```python
from build123d import *

# Parameters (mm, degrees)
LID_PLATE_START                    = 32.5
LID_FOOTPRINT_W                    = 134.2
LID_FOOTPRINT_H                    = 68.4
LID_PLATE_DEPTH                    = 3
WHEEL_CLEARANCE_WINDOWS_START      = 36
WHEEL_WELL_PROFILE_W               = 21.2
WHEEL_WELL_PROFILE_H               = 46.2
WHEEL_CLEARANCE_WINDOWS_DEPTH      = 5
LID_STIFFENING_RIBS_START          = 29.5
LID_RIB_PROFILE_W                  = 78
LID_RIB_PROFILE_H                  = 2.5
LID_STIFFENING_RIBS_DEPTH          = 3
LID_MOTOR_CLAMP_BLOCKS_START       = 23.6
UPPER_MOTOR_CLAMP_PROFILE_W        = 10
UPPER_MOTOR_CLAMP_PROFILE_H        = 19
LID_MOTOR_CLAMP_BLOCKS_DEPTH       = 8.9
UPPER_MOTOR_CLAMP_SEATS_R8P2_START = 36
UPPER_CLAMP_RADIUS_PROFILE_R       = 8.2
UPPER_MOTOR_CLAMP_SEATS_R8P2_DEPTH = 72
REGISTRATION_TABS_START            = 31
LID_REGISTRATION_PROFILE_W         = 32
LID_REGISTRATION_PROFILE_H         = 0.9
REGISTRATION_TABS_DEPTH            = 1.5
BATTERY_SOFT_PAD_STOPS_START       = 21.1
BATTERY_UPPER_STOP_PROFILE_W       = 8
BATTERY_UPPER_STOP_PROFILE_H       = 8
BATTERY_SOFT_PAD_STOPS_DEPTH       = 11.4
LID_M3_CLEARANCE_HOLES_START       = 36
LID_M3_CLEARANCE_PROFILE_R         = 1.7
LID_M3_CLEARANCE_HOLES_DEPTH       = 5
SWITCH_RETENTION_RAILS_START       = 18.4
SWITCH_RETENTION_RAIL_PROFILE_W    = 1.7
SWITCH_RETENTION_RAIL_PROFILE_H    = 8.3
SWITCH_RETENTION_RAILS_DEPTH       = 14.1
SWITCH_RETENTION_LEDGES_START      = 17.4
SWITCH_RETENTION_LEDGE_PROFILE_W   = 2.7
SWITCH_RETENTION_LEDGE_PROFILE_H   = 8.3
SWITCH_RETENTION_LEDGES_DEPTH      = 1
SWITCH_TOOL_ACCESS_START           = 36
SWITCH_TOOL_ACCESS_PROFILE_R       = 3.25
SWITCH_TOOL_ACCESS_DEPTH           = 5
LID_OUTER_CORNERS_R4_R             = 4
SNAKE_LOGO_ENGRAVED_START          = 35.5
SNAKE_LOGO_ENGRAVED_DEPTH          = 0.4


with BuildPart() as part:
    # Lid_Footprint → Lid_Plate (new body)
    with BuildSketch(Plane.XY.offset(LID_PLATE_START)):
        Rectangle(LID_FOOTPRINT_W, LID_FOOTPRINT_H)
    extrude(amount=LID_PLATE_DEPTH)

    # Wheel_Well_Profile → Wheel_Clearance_Windows (cut)
    with BuildSketch(Plane.XY.offset(WHEEL_CLEARANCE_WINDOWS_START)):
        with Locations((53.5, 0)):
            Rectangle(WHEEL_WELL_PROFILE_W, WHEEL_WELL_PROFILE_H)
        with Locations((-53.5, 0)):
            Rectangle(WHEEL_WELL_PROFILE_W, WHEEL_WELL_PROFILE_H)
    extrude(amount=-WHEEL_CLEARANCE_WINDOWS_DEPTH, mode=Mode.SUBTRACT)

    # Lid_Rib_Profile → Lid_Stiffening_Ribs (add)
    with BuildSketch(Plane.XY.offset(LID_STIFFENING_RIBS_START)):
        with Locations((0, -6.75)):
            Rectangle(LID_RIB_PROFILE_W, LID_RIB_PROFILE_H)
        with Locations((0, 6.75)):
            Rectangle(LID_RIB_PROFILE_W, LID_RIB_PROFILE_H)
    extrude(amount=LID_STIFFENING_RIBS_DEPTH)

    # Upper_Motor_Clamp_Profile → Lid_Motor_Clamp_Blocks (add)
    with BuildSketch(Plane.XY.offset(LID_MOTOR_CLAMP_BLOCKS_START)):
        with Locations((-30.1, 0)):
            Rectangle(UPPER_MOTOR_CLAMP_PROFILE_W, UPPER_MOTOR_CLAMP_PROFILE_H)
        with Locations((30.1, 0)):
            Rectangle(UPPER_MOTOR_CLAMP_PROFILE_W, UPPER_MOTOR_CLAMP_PROFILE_H)
    extrude(amount=LID_MOTOR_CLAMP_BLOCKS_DEPTH)

    # Upper_Clamp_Radius_Profile → Upper_Motor_Clamp_Seats_R8p2 (cut)
    with BuildSketch(Plane(origin=(0, 0, 0), x_dir=(0, 0, -1), z_dir=(1, 0, 0)).offset(UPPER_MOTOR_CLAMP_SEATS_R8P2_START)):
        with Locations((-19.6, 0)):
            Circle(UPPER_CLAMP_RADIUS_PROFILE_R)
    extrude(amount=-UPPER_MOTOR_CLAMP_SEATS_R8P2_DEPTH, mode=Mode.SUBTRACT)

    # Lid_Registration_Profile → Registration_Tabs (add)
    with BuildSketch(Plane.XY.offset(REGISTRATION_TABS_START)):
        with Locations((-16.5, 30.45)):
            Rectangle(LID_REGISTRATION_PROFILE_W, LID_REGISTRATION_PROFILE_H)
        with Locations((16.5, 30.45)):
            Rectangle(LID_REGISTRATION_PROFILE_W, LID_REGISTRATION_PROFILE_H)
        with Locations((-16.5, -30.45)):
            Rectangle(LID_REGISTRATION_PROFILE_W, LID_REGISTRATION_PROFILE_H)
        with Locations((16.5, -30.45)):
            Rectangle(LID_REGISTRATION_PROFILE_W, LID_REGISTRATION_PROFILE_H)
    extrude(amount=REGISTRATION_TABS_DEPTH)

    # Battery_Upper_Stop_Profile → Battery_Soft_Pad_Stops (add)
    with BuildSketch(Plane.XY.offset(BATTERY_SOFT_PAD_STOPS_START)):
        with Locations((-11, 21)):
            Rectangle(BATTERY_UPPER_STOP_PROFILE_W, BATTERY_UPPER_STOP_PROFILE_H)
        with Locations((11, 21)):
            Rectangle(BATTERY_UPPER_STOP_PROFILE_W, BATTERY_UPPER_STOP_PROFILE_H)
    extrude(amount=BATTERY_SOFT_PAD_STOPS_DEPTH)

    # Lid_M3_Clearance_Profile → Lid_M3_Clearance_Holes (cut)
    with BuildSketch(Plane.XY.offset(LID_M3_CLEARANCE_HOLES_START)):
        with Locations(Location((-52, -28.5, 0), (0, 0, 180))):
            Circle(LID_M3_CLEARANCE_PROFILE_R)
        with Locations(Location((-52, 28.5, 0), (0, 0, 180))):
            Circle(LID_M3_CLEARANCE_PROFILE_R)
        with Locations(Location((52, -28.5, 0), (0, 0, 180))):
            Circle(LID_M3_CLEARANCE_PROFILE_R)
        with Locations(Location((52, 28.5, 0), (0, 0, 180))):
            Circle(LID_M3_CLEARANCE_PROFILE_R)
    extrude(amount=-LID_M3_CLEARANCE_HOLES_DEPTH, mode=Mode.SUBTRACT)

    # Switch_Retention_Rail_Profile → Switch_Retention_Rails (add)
    with BuildSketch(Plane.XY.offset(SWITCH_RETENTION_RAILS_START)):
        with Locations((-10.65, -14.35)):
            Rectangle(SWITCH_RETENTION_RAIL_PROFILE_W, SWITCH_RETENTION_RAIL_PROFILE_H)
        with Locations((10.65, -14.35)):
            Rectangle(SWITCH_RETENTION_RAIL_PROFILE_W, SWITCH_RETENTION_RAIL_PROFILE_H)
    extrude(amount=SWITCH_RETENTION_RAILS_DEPTH)

    # Switch_Retention_Ledge_Profile → Switch_Retention_Ledges (add)
    with BuildSketch(Plane.XY.offset(SWITCH_RETENTION_LEDGES_START)):
        with Locations((-10.15, -14.35)):
            Rectangle(SWITCH_RETENTION_LEDGE_PROFILE_W, SWITCH_RETENTION_LEDGE_PROFILE_H)
        with Locations((10.15, -14.35)):
            Rectangle(SWITCH_RETENTION_LEDGE_PROFILE_W, SWITCH_RETENTION_LEDGE_PROFILE_H)
    extrude(amount=SWITCH_RETENTION_LEDGES_DEPTH)

    # Switch_Tool_Access_Profile → Switch_Tool_Access (cut)
    with BuildSketch(Plane.XY.offset(SWITCH_TOOL_ACCESS_START)):
        with Locations(Location((3.175, -14.325, 0), (0, 0, 180))):
            Circle(SWITCH_TOOL_ACCESS_PROFILE_R)
    extrude(amount=-SWITCH_TOOL_ACCESS_DEPTH, mode=Mode.SUBTRACT)

    # Lid_Outer_Corners_R4
    lid_outer_corners_r4_edges = [part.edges().sort_by_distance(p)[0] for p in [
        (-67.1, 34.2, 34),
        (67.1, 34.2, 34),
        (67.1, -34.2, 34),
        (-67.1, -34.2, 34),
    ]]
    fillet(lid_outer_corners_r4_edges, radius=LID_OUTER_CORNERS_R4_R)

    # Snake_Logo_Native_Profile → Snake_Logo_Engraved (cut)
    # profile 1 of 2: a face of its own
    with BuildSketch(Plane.XY.offset(SNAKE_LOGO_ENGRAVED_START)):
        Polygon((13.800582242, 26.557496361), (14.851528384, 25.064046579), (14.851528384, 24.898107715), (6.443959243, 19.311499272), (14.243085881, 18.703056769), (15.459970888, 22.851528384), (15.625909753, 23.349344978), (15.791848617, 23.459970888), (19, 17.983988355), (9.430858806, 12.010189229), (4.397379913, -0.767103348), (4.065502183, -1.320232897), (5.890829694, 11.45705968), (0.027656477, 13.890829694), (-5.890829694, 11.45705968), (-4.065502183, -0.877729258), (-4.065502183, -1.264919942), (-4.176128093, -1.320232897), (-9.430858806, 12.010189229), (-19, 17.983988355), (-15.791848617, 23.459970888), (-15.570596798, 23.183406114), (-14.243085881, 18.703056769), (-6.443959243, 19.311499272), (-14.851528384, 24.898107715), (-14.851528384, 25.064046579), (-13.911208151, 26.502183406), (-0.414847162, 24.84279476), (0.414847162, 24.84279476), align=None)
        Polygon((-4.452692868, 14.720524017), (-2.018922853, 14.775836972), (-3.788937409, 16.490538574), align=None, mode=Mode.SUBTRACT)
        Polygon((1.963609898, 14.720524017), (4.452692868, 14.720524017), (3.788937409, 16.490538574), align=None, mode=Mode.SUBTRACT)
    # profile 2 of 2: a face of its own
    with BuildSketch(Plane.XY.offset(SNAKE_LOGO_ENGRAVED_START)):
        Polygon((-16.84279476, 15.107714702), (-16.566229985, 15.052401747), (-16.62154294, 14.941775837), (-16.510917031, 14.997088792), (-15.902474527, 14.554585153), (-13.136826783, 12.397379913), (-13.026200873, 12.176128093), (-6.775836972, -5.855895197), (-3.788937409, -6.740902475), (-3.180494905, -4.141193595), (-3.014556041, -4.08588064), (-2.240174672, -7.183406114), (-0.082969432, -7.847161572), (2.240174672, -7.128093159), (3.014556041, -4.141193595), (3.180494905, -4.19650655), (3.788937409, -6.740902475), (6.775836972, -5.855895197), (13.081513828, 12.342066958), (16.62154294, 15.107714702), (16.787481805, 14.997088792), (13.800582242, 12.010189229), (7.937409025, -7.625909753), (0.304221252, -10.502183406), (-0.138282387, -10.557496361), (-7.937409025, -7.625909753), (-13.800582242, 12.010189229), align=None)
    extrude(amount=-SNAKE_LOGO_ENGRAVED_DEPTH, mode=Mode.SUBTRACT)


solid = part.part
```
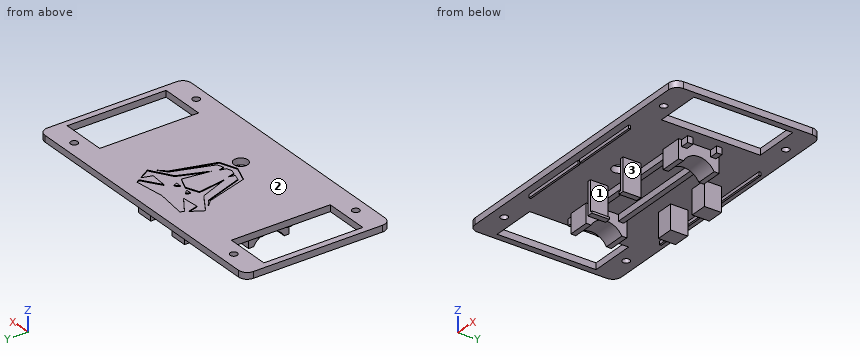
The model under review builds one solid part; all positions refer to its coordinate system, in mm. Face numbers are marked on the shaded views. Round coordinates to 2 decimals unless told otherwise and drop trailing zeros. Loops run counter-clockwise (first coordinate to the right, second up) from the corner with the lowest first, then second, coordinate; pieces in that order, holes last. Notation, with made-up numbers: (-25, -39) - (29, -39) arc R27 cw to (29, -9) - close; hole circle Ø6 at (-38.75, 4). An arc over 180 degrees is marked (long way). Use a Markdown table: item, result. Add a question column.
Q1. Add section D-D (x = -47.5). State the section outline as (y, z) points, plus the area to 3 significant figures.
Q2. For probe 1 along X at (y, z) = (28.5, 33.85); probe 2 along X at (y, z) = (3, 34.5); probe 3 along Y at (x, z) = (-52, 33.7), list the stretches that pass through material, from the lowest coordinate up.
Q3. Insertion check: pin 1 Ø1.2 at (x, z) = (17, 32) entering from -Y; pin 2 Ø0.8 at (x, z) = (-14.5, 31.5) entering from +Y; pin 3 Ø5 at (x, y) = (-10, 15.5) entering from +Z; pin 4 Ø2 at (x, y) = (36, 7) entering from -Z. Each pin has a flat end and moves straight along its axis. Give the tip position at first contact, or say it passes through.
Q4. Add section C-C (x = 23.5). State the section outline as (y, z) points, plus the area to 3 significant figures.
Q5. Add section A-A (y = -28.5). State the section outline as (x, z) points.
Q6. The part is to be moulded in two halves that separate along X. For the marked faces 1, 2 and 3, say which applies: pulls with the +X half, pulls with the -X half, needs draft (parallel to the pull), parting line crosses it, or undercut.
Q7. Add section B-B (x = 52). State the section outline as (y, z) points.
Worked answers:
| question | item | result |
|---|---|---|
| 1 | outline | (-34.2, 32.5) - (-23.1, 32.5) - (-23.1, 35.5) - (-34.2, 35.5) - close; (23.1, 32.5) - (34.2, 32.5) - (34.2, 35.5) - (23.1, 35.5) - close |
| 1 | area | 66.6 mm² |
| 2 | probe 1 | -67.1 to -53.7, -50.3 to 50.3, 53.7 to 67.1 |
| 2 | probe 2 | -67.1 to -64.1, -42.9 to 42.9, 64.1 to 67.1 |
| 2 | probe 3 | -34.2 to -30.2, -26.8 to -23.1, 23.1 to 26.8, 30.2 to 34.2 |
| 3 | pin 1 | y = -34.2 |
| 3 | pin 2 | y = 30.9 |
| 3 | pin 3 | z = 35.1 |
| 3 | pin 4 | z = 23.6 |
| 4 | outline | (-34.2, 32.5) - (-30.9, 32.5) - (-30.9, 31) - (-30, 31) - (-30, 32.5) - (-8, 32.5) - (-8, 29.5) - (-5.5, 29.5) - (-5.5, 32.5) - (5.5, 32.5) - (5.5, 29.5) - (8, 29.5) - (8, 32.5) - (30, 32.5) - (30, 31) - (30.9, 31) - (30.9, 32.5) - (34.2, 32.5) - (34.2, 35.5) - (-34.2, 35.5) - close |
| 4 | area | 223 mm² |
| 5 | outline | (-67.1, 32.5) - (-53.7, 32.5) - (-53.7, 35.5) - (-67.1, 35.5) - close; (-50.3, 32.5) - (50.3, 32.5) - (50.3, 35.5) - (-50.3, 35.5) - close; (53.7, 32.5) - (67.1, 32.5) - (67.1, 35.5) - (53.7, 35.5) - close |
| 6 | face 1 | undercut |
| 6 | face 2 | needs draft |
| 6 | face 3 | pulls with the +X half |
| 7 | outline | (-34.2, 32.5) - (-30.2, 32.5) - (-30.2, 35.5) - (-34.2, 35.5) - close; (-26.8, 32.5) - (-23.1, 32.5) - (-23.1, 35.5) - (-26.8, 35.5) - close; (23.1, 32.5) - (26.8, 32.5) - (26.8, 35.5) - (23.1, 35.5) - close; (30.2, 32.5) - (34.2, 32.5) - (34.2, 35.5) - (30.2, 35.5) - close |
